Read the model definition and answer for the solid it produces. Units are mm, in the model's axes. A direction names the side the tool comes from. Round coordinates to 2 decimals unless told otherwise and drop trailing zeros. Write each loop counter-clockwise with the first axis right and the second up, starting at its lowest first coordinate (ties: lowest second). Pieces come first, ordered by that corner, then holes.
from build123d import *

# Parameters (mm, degrees)
SKETCH_1_R               = 6
EXTRUDE_1_DEPTH          = 2.5
SKETCH_2_R               = 4
EXTRUDE_2_DEPTH          = 25
CUT_EXTRUDE_1_DEPTH      = 29.779332862
CUT_EXTRUDE_1_DEPTH_BACK = 29.779332862
SKETCH_3_R               = 1.6


with BuildPart() as part:
    # 草图1 → 凸台-拉伸1 (new body)
    with BuildSketch(Plane(origin=(0, 0, 0), x_dir=(1, 0, 0), z_dir=(0, 1, 0))):
        with Locations(Location((0, 0, 0), (0, 0, 270))):
            Circle(SKETCH_1_R)
    extrude(amount=EXTRUDE_1_DEPTH)

    # 草图2 → 凸台-拉伸2 (add)
    with BuildSketch(Plane(origin=(0, 2.5, 0), x_dir=(1, 0, 0), z_dir=(0, 1, 0))):
        with Locations(Location((0, 0, 0), (0, 0, 270))):
            Circle(SKETCH_2_R)
    extrude(amount=EXTRUDE_2_DEPTH)

    # 草图3 → 切除-拉伸1 (cut, two sides: drawn at the far end of the back side and taken through both)
    with BuildSketch(Plane(origin=(0, 0, 0), x_dir=(0, 0, -1), z_dir=(1, 0, 0)).offset(-CUT_EXTRUDE_1_DEPTH_BACK)):
        with Locations((0, 23.5)):
            Circle(SKETCH_3_R)
    extrude(amount=CUT_EXTRUDE_1_DEPTH + CUT_EXTRUDE_1_DEPTH_BACK, mode=Mode.SUBTRACT)


solid = part.part
Q1. Section A-A (z = 0) is taken. Determine the outline of the cut face in (x, y), then the cut area to 3 significant figures.
Verdict:
outline: (-6, 0) - (6, 0) - (6, 2.5) - (4, 2.5) - (4, 21.9) - (-4, 21.9) - (-4, 2.5) - (-6, 2.5) - close; (-4, 25.1) - (4, 25.1) - (4, 27.5) - (-4, 27.5) - close
area: 204 mm2
Q2. Flat-ended cylindrical pins translate along their axes: pin 1 Ø5 at (y, z) = (23.5, 0) entering from +X; pin 2 Ø5 at (x, y) = (2, 24) entering from +Z; pin 3 Ø6 at (x, y) = (2.5, 24.5) entering from -Z. Find the tip coordinate at first contact, or state that the pin passes through.
Verdict:
pin 1: stops at x = 4
pin 2: stops at z = 4
pin 3: stops at z = -4
Q3. Section B-B (x = 0) is taken. Determine the outline of the cut face in (y, z), then the cut area to 3 significant figures.
Verdict:
outline: (0, -6) - (2.5, -6) - (2.5, -4) - (27.5, -4) - (27.5, 4) - (2.5, 4) - (2.5, 6) - (0, 6) - close; hole circle Ø3.2 at (23.5, 0)
area: 222 mm2
Q4. Determine the mould class of faces 1 (the flat face through (0, 0, 0)), 2 (the flat face through (0, 27.5, 0)), 3 (the cylindrical face through (-0.056, 25.086, 0.208)) for opening direction Y: pulls with the +Y half, pulls with the -Y half, needs draft (parallel to the pull), parting line crosses it, or undercut.
Verdict:
face 1: pulls with the -Y half
face 2: pulls with the +Y half
face 3: undercut
Q5. Section C-C (y = 13) is taken. Determine the outline of the cut face in (x, z).
Verdict:
outline: circle Ø8 at (0, 0)
Q6. Straight lines are drawn through the part: probe 1 along Y at (x, z) = (1, 0); probe 2 along Y at (x, z) = (0.5, 1); probe 3 along Z at (x, y) = (2, 23.5). For each, find the intervals that lie inside material, in ascending order.
Verdict:
probe 1: y = 0 to 21.9, 25.1 to 27.5
probe 2: y = 0 to 22.25, 24.75 to 27.5
probe 3: z = -3.46 to -1.6, 1.6 to 3.46
Q7. Which of the six approach directions +Z, -Z, +X, -X, +Y, -Y give full straight-line access (tool end or side, diameter ignored) to faces 4 (the flat face through (-3.92, 2.5, -1.42)), 5 (the cylindrical face through (1.802, 1.232, 5.723))?
Verdict:
face 4: +Y
face 5: +Y, -Y
Q8. Section D-D (z = 2.5) is taken. Determine the outline of the cut face in (x, y).
Verdict:
outline: (-5.45, 0) - (5.45, 0) - (5.45, 2.5) - (3.12, 2.5) - (3.12, 27.5) - (-3.12, 27.5) - (-3.12, 2.5) - (-5.45, 2.5) - close
